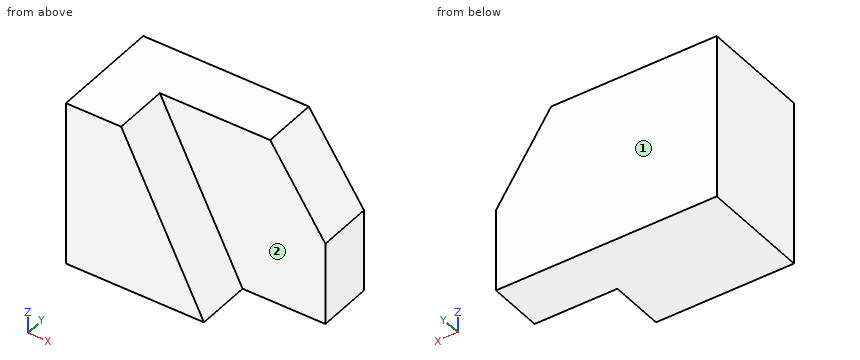
from build123d import *

# Parameters (mm, degrees)
F0_W     = 101.6
F0_H     = 76.2
F1_DEPTH = 50.8
F3_DEPTH = 25.4
F5_DEPTH = 25.4


with BuildPart() as f1:
    # F0 (on Front) → F1 (new body)
    with BuildSketch(Plane.XZ):
        Rectangle(F0_W, F0_H)
    extrude(amount=F1_DEPTH)

    # F2 (on face) → F3 (cut)
    with BuildSketch(Plane.XZ.offset(50.8)):
        Polygon((50.8, 38.1), (-25.4, 38.1), (12.7, -38.1), (50.8, -38.1), align=None)
    extrude(amount=-F3_DEPTH, mode=Mode.SUBTRACT)

    # F4 (on face) → F5 (cut)
    with BuildSketch(Plane.XZ.offset(25.4)):
        Polygon((50.8, 38.1), (25.4, 38.1), (50.8, 0), align=None)
    extrude(amount=-F5_DEPTH, mode=Mode.SUBTRACT)


solid = f1.part
Part model, mm, in its own coordinate system. Face numbers are marked on the shaded views. A direction names the side the tool comes from. Coordinates: 2 decimals unless noted, no trailing zeros. Write each loop counter-clockwise with the first axis right and the second up, starting at its lowest first coordinate (ties: lowest second). Pieces come first, ordered by that corner, then holes. Notation, with made-up numbers: M 69,7 L 97,7 A27 ccw 97,41 Z; hole C 26,55 d5. An arc over 180 degrees is marked long. Return JSON: item names as keys, results as strings.
1. Flat gauge pins, fed straight in: pin 1 Ø4 at (y, z) = (-35, -16.5) entering from +X; pin 2 Ø5 at (y, z) = (-34, -2) entering from +X. Where does each tip first touch, or does it go through?
Determined:
{"pin 1": "x = 2.9", "pin 2": "x = -4.1"}
2. Saw through at D-D, the plane y = -13. Write the cut outline in (x, z).
Determined:
{"outline": "M -50.8,-38.1 L 50.8,-38.1 L 50.8,0 L 25.4,38.1 L -50.8,38.1 Z"}
3. Saw through at A-A, the plane z = -32.5. Write the cut outline in (x, y).
Determined:
{"outline": "M -50.8,-50.8 L 9.9,-50.8 L 9.9,-25.4 L 50.8,-25.4 L 50.8,0 L -50.8,0 Z"}
4. Probe L1, parallel to Y at x = 37, z = -15.5; L2, parallel to Z at x = -13, y = -44.5; L3, parallel to Z at x = 42, y = -3. List the from-to ranges inside material, lowest first.
Determined:
{"L1": "-25.4 to 0", "L2": "-38.1 to 13.3", "L3": "-38.1 to 13.2"}
5. 3-axis set-ups, long thin cutter, end or side, ignore diameter. For the marked faces 1 and 2: which of +Z, -Z, +X, -X, +Y, -Y reach the whole face in a straight line?
Determined:
{"face 1": "+Z, -Z, +X, -X, +Y", "face 2": "+Z, +X, -Y"}
6. Saw through at C-C, the plane y = -46. Write the cut outline in (x, z), then the cut area to 3 significant figures.
Determined:
{"outline": "M -50.8,-38.1 L 12.7,-38.1 L -25.4,38.1 L -50.8,38.1 Z", "area": "3,390 mm²"}
7. Saw through at B-B, the plane x = -12.5. Write the cut outline in (y, z).
Determined:
{"outline": "M -50.8,-38.1 L 0,-38.1 L 0,38.1 L -25.4,38.1 L -25.4,12.3 L -50.8,12.3 Z"}
